from build123d import *

# Parameters (mm, degrees)
F0_R     = 75
F1_DEPTH = 3
F2_R     = 75
F2_R_2   = 71
F3_DEPTH = 55
F4_R     = 5
F4_R_2   = 1.5
F5_DEPTH = 50


with BuildPart() as f1:
    # F0 (on Top) → F1 (new body)
    with BuildSketch(Plane.XY):
        Circle(F0_R)
    extrude(amount=F1_DEPTH)

    # F2 (on face) → F3 (join)
    with BuildSketch(Plane.XY.offset(3)):
        Circle(F2_R)
        Circle(F2_R_2, mode=Mode.SUBTRACT)
    extrude(amount=F3_DEPTH)

    # F4 (on face) → F5 (join)
    with BuildSketch(Plane.XY.offset(3)):
        with Locations((0, 67.343959)):
            Circle(F4_R)
        with Locations((0, 67.343959)):
            Circle(F4_R_2, mode=Mode.SUBTRACT)
        with Locations((-67.343959, 0)):
            Circle(F4_R)
        with Locations((-67.343959, 0)):
            Circle(F4_R_2, mode=Mode.SUBTRACT)
        with Locations((0, -67.343959)):
            Circle(F4_R)
        with Locations((0, -67.343959)):
            Circle(F4_R_2, mode=Mode.SUBTRACT)
        with Locations((67.343959, 0)):
            Circle(F4_R)
        with Locations((67.343959, 0)):
            Circle(F4_R_2, mode=Mode.SUBTRACT)
    extrude(amount=F5_DEPTH)


solid = f1.part
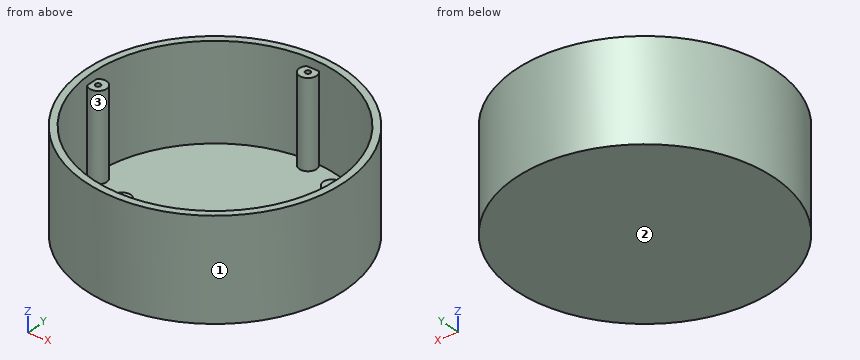
Work out the finished part from the listing and answer in its coordinate system (mm). Face numbers are marked on the shaded views. Coordinates: 2 decimals unless noted, no trailing zeros. Loops run counter-clockwise (first coordinate to the right, second up) from the corner with the lowest first, then second, coordinate; pieces in that order, holes last. Notation, with made-up numbers: M 50.25,59.25 L 54.25,59.25 A21 cw 54.25,85.25 Z; hole C -34,-19 d7. An arc over 180 degrees is marked long. Answer in a Markdown table with one row per item. Add a question column.
1. Consider L1, parallel to Y at x = -4, z = 49; L2, parallel to Y at x = 0, z = 31.5; L3, parallel to Z at x = -44, y = 3.5. Determine where each line is inside the solid, lowest interval first.
2. The mould has two halves that part along X. Classify the marked faces 1, 2 and 3: pulls with the +X half, pulls with the -X half, needs draft (parallel to the pull), parting line crosses it, or undercut.
3. Find section C-C, the plane y = -13.5. Write down the section's boundary in (x, z) (3 decimals), then the cut area to 3 significant figures.
4. Flat-ended cylindrical pins translate along their axes: P1, Ø1.5, axis at x = 30, z = 26.5, coming from the -Y side; P2, Ø5, axis at y = -12.5, z = 19.5, coming from the -X side; P3, Ø12, axis at y = 45.5, z = 20.5, coming from the -X side. Find the tip coordinate at first contact, or state that the pin passes through.
5. Find section A-A, the plane x = 48. Write down the section's boundary in (y, z), then the cut area to 3 significant figures.
6. Find section B-B, the plane z = 32.5. Write down the section's boundary in (x, y).
Reported:
| question | item | result |
|---|---|---|
| 1 | L1 | y = -74.89 to -70.89, -70.34 to -64.34, 64.34 to 70.34, 70.89 to 74.89 |
| 1 | L2 | y = -75 to -68.84, -65.84 to -62.34, 62.34 to 65.84, 68.84 to 75 |
| 1 | L3 | z = 0 to 3 |
| 2 | face 1 | parting line crosses it |
| 2 | face 2 | needs draft |
| 2 | face 3 | undercut |
| 3 | outline | M -73.775,0 L 73.775,0 L 73.775,58 L 69.705,58 L 69.705,3 L -69.705,3 L -69.705,58 L -73.775,58 Z |
| 3 | area | 890 mm^2 |
| 4 | P1 | stops at y = -69.06 |
| 4 | P2 | stops at x = -74.33 |
| 4 | P3 | stops at x = -63.76 |
| 5 | outline | M -57.63,0 L 57.63,0 L 57.63,58 L 52.32,58 L 52.32,3 L -52.32,3 L -52.32,58 L -57.63,58 Z |
| 5 | area | 930 mm^2 |
| 6 | outline | C 0,0 d150; hole M -70.91,-3.5 A71 ccw -3.5,-70.91 A5 cw long 3.5,-70.91 A71 ccw 70.91,-3.5 A5 cw long 70.91,3.5 A71 ccw 3.5,70.91 A5 cw long -3.5,70.91 A71 ccw -70.91,3.5 A5 cw long Z; hole C -67.34,0 d3; hole C 0,-67.34 d3; hole C 0,67.34 d3; hole C 67.34,0 d3 |
